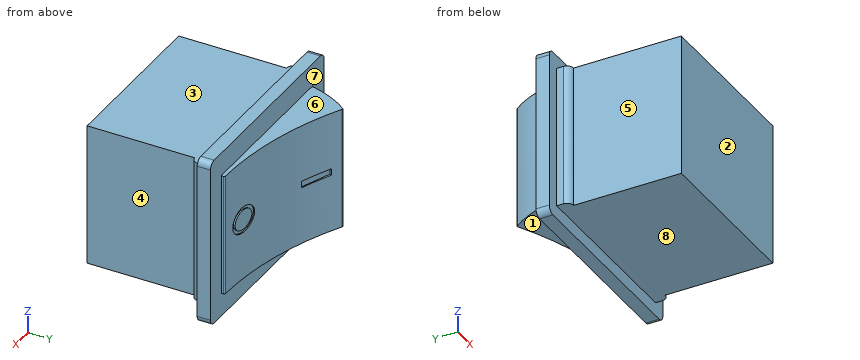
from build123d import *

# Parameters (mm, degrees)
CROQUIS1_W                   = 31
CROQUIS1_H                   = 25.5
CROQUIS1_W_2                 = 25
CROQUIS1_H_2                 = 18.5
SALIENTE_EXTRUIR1_DEPTH      = 2
REDONDEO1_R                  = 1
CROQUIS2_W                   = 25
CROQUIS2_H                   = 21.5
SALIENTE_EXTRUIR5_DEPTH      = 18.2
SALIENTE_EXTRUIR5_DEPTH_BACK = 1
SALIENTE_EXTRUIR6_DEPTH      = 10.75
SALIENTE_EXTRUIR7_DEPTH      = 9.2
CROQUIS7_RX                  = 2.5
CROQUIS7_RY                  = 1.989859087
CROQUIS7_RX_2                = 1.919157188
CROQUIS7_RY_2                = 1.506996734
CROQUIS7_W                   = 5
CROQUIS7_H                   = 1
CORTAR_EXTRUIR2_DEPTH        = 0.5
CROQUIS8_RX                  = 2.5
CROQUIS8_RY                  = 1.989859087
CROQUIS8_RX_2                = 1.919157188
CROQUIS8_RY_2                = 1.506996734
CROQUIS8_W                   = 5
CROQUIS8_H                   = 1
CORTAR_EXTRUIR3_DEPTH        = 0.5


with BuildPart() as part:
    # Croquis1 → Saliente-Extruir1 (new body)
    with BuildSketch(Plane(origin=(0, 0, 0), x_dir=(1, 0, 0), z_dir=(0, 1, 0))):
        Rectangle(CROQUIS1_W, CROQUIS1_H)
        Rectangle(CROQUIS1_W_2, CROQUIS1_H_2, mode=Mode.SUBTRACT)
    extrude(amount=SALIENTE_EXTRUIR1_DEPTH)

    # Redondeo1
    redondeo1_edges = [part.edges().sort_by_distance(p)[0] for p in [
        (15.5, 1, 12.75),
        (-15.5, 1, 12.75),
        (-15.5, 1, -12.75),
        (15.5, 1, -12.75),
    ]]
    fillet(redondeo1_edges, radius=REDONDEO1_R)

    # Croquis2 → Saliente-Extruir5 (add, two sides)
    with BuildSketch(Plane.XZ) as saliente_extruir5_sk:
        Rectangle(CROQUIS2_W, CROQUIS2_H)
    extrude(amount=SALIENTE_EXTRUIR5_DEPTH)
    extrude(saliente_extruir5_sk.sketch, amount=-SALIENTE_EXTRUIR5_DEPTH_BACK)

    # Croquis3 → Saliente-Extruir6 (add, symmetric)
    with BuildSketch(Plane.XY):
        with BuildLine():
            Line((12.5, 0), (13.5, 0))
            Line((13.5, 0), (13.5, -1))
            ThreePointArc((13.5, -1), (13.207106781, -1.707106781), (12.5, -2))
            Line((12.5, -2), (12.5, 0))
        make_face()
        with BuildLine():
            Line((-12.5, 0), (-12.5, -2))
            ThreePointArc((-12.5, -2), (-13.207106781, -1.707106781), (-13.5, -1))
            Line((-13.5, -1), (-13.5, 0))
            Line((-13.5, 0), (-12.5, 0))
        make_face()
    extrude(amount=SALIENTE_EXTRUIR6_DEPTH, both=True)

    # Croquis4 → Saliente-Extruir7 (add, symmetric)
    with BuildSketch(Plane.XY):
        with BuildLine():
            ThreePointArc((-9.347385872, 8.117762074), (1.152636372, 4.009298277), (12.326652836, 2.502215681))
            ThreePointArc((12.326652836, 2.502215681), (12.45734879, 2.45105267), (12.522240679, 2.326601358))
            ThreePointArc((12.522240679, 2.326601358), (12.589620665, 1.664412167), (12.62950875, 1))
            ThreePointArc((12.62950875, 1), (0.064754375, -1.4616694), (-12.5, 1))
            ThreePointArc((-12.5, 1), (-11.477075864, 4.704087901), (-9.603642409, 8.059216522))
            ThreePointArc((-9.603642409, 8.059216522), (-9.48648288, 8.136499966), (-9.347385872, 8.117762074))
        make_face()
    extrude(amount=SALIENTE_EXTRUIR7_DEPTH, both=True)

    # Croquis7 → Cortar-Extruir2 (cut, symmetric)
    with BuildSketch(Plane(origin=(1.513513313, 3.868093829, 0), x_dir=(-0.93125002, 0.364380846, 0), z_dir=(-0.364380846, -0.93125002, 0))):
        with Locations(Location((-7.5, 0), (0, 0, -180))):
            Ellipse(CROQUIS7_RX, CROQUIS7_RY)
        with Locations(Location((-7.5, 0), (0, 0, -180))):
            Ellipse(CROQUIS7_RX_2, CROQUIS7_RY_2, mode=Mode.SUBTRACT)
        with Locations((7.5, 0)):
            Rectangle(CROQUIS7_W, CROQUIS7_H)
    extrude(amount=CORTAR_EXTRUIR2_DEPTH, both=True, mode=Mode.SUBTRACT)

    # Croquis8 → Cortar-Extruir3 (cut, symmetric)
    with BuildSketch(Plane(origin=(0.55168143, 4.090351383, 0), x_dir=(-0.991026762, 0.133663593, 0), z_dir=(-0.133663593, -0.991026762, 0))):
        with Locations(Location((-7.5, 0), (0, 0, -180))):
            Ellipse(CROQUIS8_RX, CROQUIS8_RY)
        with Locations(Location((-7.5, 0), (0, 0, -180))):
            Ellipse(CROQUIS8_RX_2, CROQUIS8_RY_2, mode=Mode.SUBTRACT)
        with Locations((7.5, 0)):
            Rectangle(CROQUIS8_W, CROQUIS8_H)
    extrude(amount=CORTAR_EXTRUIR3_DEPTH, both=True, mode=Mode.SUBTRACT)


solid = part.part
The model under review builds one solid part; all positions refer to its coordinate system, in mm. Face numbers are marked on the shaded views. A direction names the side the tool comes from. Give positions to 0.01 mm unless a question says otherwise; leave off trailing zeros. Order: outer loops, then holes, each group sorted by start corner. A loop starts at its lowest first (then second) coordinate and runs counter-clockwise, first axis right, second up. Notation, with made-up numbers: M -35.5,62.5 L 18.5,62.5 A26 ccw 18.5,97.5 Z; hole C 0.5,1.5 d8. An arc over 180 degrees is marked long. Use one line per item in the form item = value. Start each with the question number.
Item 1: To check wall thickness, follow line 1 along Z through (x, y) = (-7, -0.5); line 2 along X through (y, z) = (-10.75, -4.75); line 3 along Y through (x, z) = (-7.5, 11.25). State the ranges of each line that lie inside material, in increasing order. Write a range as from..to.
Item 2: The part is to be moulded in two halves that separate along Z. For the marked faces 6, 7 and 8, say which applies: pulls with the +Z half, pulls with the -Z half, needs draft (parallel to the pull), parting line crosses it, or undercut.
Item 3: We need section C-C on y = -5. Give the boundary of the cut face in (x, z), plus the area to 4 significant figures.
Item 4: We need section A-A on z = -6.5. Give the boundary of the cut face in (x, y).
Item 5: Insertion check: pin 1 Ø8 at (y, z) = (-7, -1.5) entering from -X; pin 2 Ø5 at (y, z) = (-12, 3) entering from +X; pin 3 Ø2 at (x, z) = (-6, 6) entering from +Y. Each pin has a flat end and moves straight along its axis. Give the tip position at first contact, or say it passes through.
Item 6: For the marked faces 1, 2, 3, 4 and 5, list the 3-axis set-ups (+Z, -Z, +X, -X, +Y, -Y) from which the entire face can be reached by the end or side of a thin tool; tool diameter is ignored.
Item 7: We need section B-B on x = 2.5. Give the boundary of the cut face in (y, z), plus the area to 3 significant figures.
Item 8: We need section D-D on x = -11.5. Give the boundary of the cut face in (y, z).
Completed:
q1.line_1 = -10.75..10.75
q1.line_2 = -12.5..12.5
q1.line_3 = 0..2
q2.face_6 = undercut
q2.face_7 = needs draft
q2.face_8 = pulls with the -Z half
q3.outline = M -12.5,-10.75 L 12.5,-10.75 L 12.5,10.75 L -12.5,10.75 Z
q3.area = 537.5 mm²
q4.outline = M -15.5,0 L -13.5,0 L -13.5,-1 A1 ccw -12.5,-2 L -12.5,-18.2 L 12.5,-18.2 L 12.5,-2 A1 ccw 13.5,-1 L 13.5,0 L 15.5,0 L 15.5,2 L 12.56,2 A16.06 ccw 12.52,2.33 A0.2 ccw 12.33,2.5 A47.31 cw -9.35,8.12 A0.2 ccw -9.6,8.06 A16.06 ccw -12.5,1 L -12.5,2 L -15.5,2 Z
q5.pin_1 = -12.5
q5.pin_2 = 12.5
q5.pin_3 = 6.94
q6.face_1 = +Y
q6.face_2 = +Z, -Z, +X, -X, -Y
q6.face_3 = +Z, +X, -X, -Y
q6.face_4 = +Z, -Z, +X, -Y
q6.face_5 = +Z, -Z, -X, -Y
q7.outline = M -18.2,-10.75 L 0,-10.75 L 0,-12.75 L 2,-12.75 L 2,-9.25 L 1,-9.25 L 1,-9.2 L 3.68,-9.2 L 3.68,9.2 L 1,9.2 L 1,9.25 L 2,9.25 L 2,12.75 L 0,12.75 L 0,10.75 L -18.2,10.75 Z
q7.area = 473 mm²
q8.outline = M -18.2,-10.75 L 0,-10.75 L 0,-12.75 L 2,-12.75 L 2,-9.25 L 1,-9.25 L 1,-9.2 L 4.65,-9.2 L 4.65,9.2 L 1,9.2 L 1,9.25 L 2,9.25 L 2,12.75 L 0,12.75 L 0,10.75 L -18.2,10.75 Z
